For this review, take the finished solid that the model builds, in its own axes (mm). Face numbers are marked on the shaded views. A direction names the side the tool comes from. Round coordinates to 2 decimals unless told otherwise and drop trailing zeros. Write each loop counter-clockwise with the first axis right and the second up, starting at its lowest first coordinate (ties: lowest second). Pieces come first, ordered by that corner, then holes. Notation, with made-up numbers: (-25, 44.25) - (28, 44.25) arc R23 cw to (28, 55.25) - close; hole circle Ø1 at (85.5, 6.25). An arc over 180 degrees is marked (long way). One line per item, written item: value. Start each with the question number.
Q1. For probe 1 along Y at (x, z) = (0, 6.6); probe 2 along Y at (x, z) = (0, 1.5); probe 3 along Z at (x, y) = (1.75, -5.75), list the stretches that pass through material, from the lowest coordinate up.
Q2. Clearance check with flat-ended pins moving along their axes: pin 1 Ø2.5 at (x, y) = (-1.5, 1.5) entering from +Z; pin 2 Ø3.5 at (x, y) = (0, 0) entering from -Z; pin 3 Ø6 at (x, z) = (7, 1.5) entering from -Y; pin 4 Ø2 at (x, z) = (-6.5, 5.5) entering from +Y. State where each tip first meets the part, or that it passes through.
Q3. Add section D-D on x = -6.25. Write out the cut boundary in (y, z).
Q4. Add section C-C on z = 7.5. Write out the cut boundary in (x, y).
Q5. Add section A-A on y = 0. Write out the cut boundary in (x, z), and give its area (3 significant figures).
Q6. Mouldability with a two-part tool opening along X and no side actions: class the marked faces 1, 2 and 3 as +X half, -X half, draft (parallel to the pull), parting line (faces both ways), or undercut.
Q7. Tool access review of the marked faces 4 and 5: name each direction out of +Z, -Z, +X, -X, +Y, -Y from which nothing blocks a thin tool from reaching the whole face with its end or side.
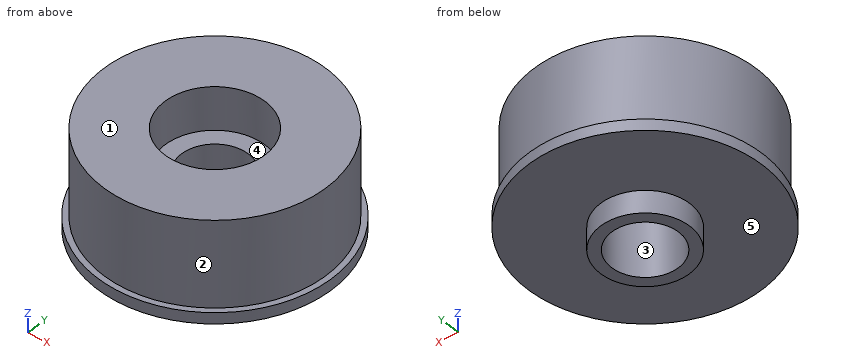
Autodesk Inventor part; units mm, degrees
ref_plane "YZ Plane" through (0, 0, 0) normal (1, 0, 0) x (0, 1, 0)
ref_plane "XZ Plane" through (0, 0, 0) normal (0, 1, 0) x (-1, 0, 0)
ref_plane "XY Plane" through (0, 0, 0) normal (0, 0, 1) x (1, 0, 0)
sketch "スケッチ1" plane through (0, 0, 0) normal (0, 0, 1) x (1, 0, 0)
  circle A0 centre (0, 0) radius 10 construction
  circle A1 centre (0, 0) radius 10.5 construction
  circle A2 centre (0, 0) radius 3 construction
  circle A3 centre (0, 0) radius 9.5 construction
  circle A4 centre (0, 0) radius 1.5
  dimension "d0" = 20
  dimension "d1" = 21
  dimension "d2" = 6
  dimension "d3" = 19
  dimension "d10" = 3
sketch "スケッチ2" plane through (0, 0, 0) normal (0, 0, 1) x (1, 0, 0)
  circle A0 centre (0, 0) radius 9.5 construction
  circle A1 centre (0, 0) radius 10 construction
  circle A2 centre (0, 0) radius 9.5
  circle A3 centre (0, 0) radius 10
extrude "押し出し1" add sketch "スケッチ2" along normal blind 8.75
sketch "スケッチ4" plane through (0, 0, 0) normal (0, 0, 1) x (1, 0, 0)
  circle A0 centre (0, 0) radius 3 construction
  circle A1 centre (0, 0) radius 9.5 construction
  circle A2 centre (0, 0) radius 9.5
  circle A3 centre (0, 0) radius 10
  circle A4 centre (0, 0) radius 3
extrude "押し出し3" add sketch "スケッチ4" along normal blind 8.75 contours A2 | A4
sketch "スケッチ6" plane through (0, 0, 0) normal (0, 0, 1) x (1, 0, 0)
  circle A0 centre (0, 0) radius 10 construction
  circle A1 centre (0, 0) radius 10.5 construction
  circle A2 centre (0, 0) radius 3 construction
  circle A3 centre (0, 0) radius 9.5 construction
  circle A4 centre (0, 0) radius 1.5
  circle A5 centre (0, 0) radius 10.5
  circle A6 centre (0, 0) radius 10
  circle A7 centre (0, 0) radius 10
  circle A8 centre (0, 0) radius 9.5
  circle A9 centre (0, 0) radius 3
  dimension "d15" = 20
  dimension "d16" = 21
  dimension "d17" = 6
  dimension "d18" = 19
  dimension "d19" = 3
extrude "押し出し6" add sketch "スケッチ6" along normal blind 1 contours A5
sketch "スケッチ7" plane through (0, 0, 0) normal (0, 0, 1) x (1, 0, 0)
  circle A0 centre (0, 0) radius 10 construction
  circle A1 centre (0, 0) radius 10.5 construction
  circle A2 centre (0, 0) radius 3 construction
  circle A3 centre (0, 0) radius 9.5 construction
  circle A4 centre (0, 0) radius 1.5
  circle A5 centre (0, 0) radius 10.5
  circle A6 centre (0, 0) radius 10
  circle A7 centre (0, 0) radius 9.5
  circle A8 centre (0, 0) radius 3
  circle A9 centre (0, 0) radius 4
  dimension "d22" = 20
  dimension "d23" = 21
  dimension "d24" = 6
  dimension "d25" = 19
  dimension "d26" = 3
  dimension "d27" = 8
extrude "押し出し7" add sketch "スケッチ7" against normal blind 2 contours A9
sketch "スケッチ8" plane through (0, 0, 0) normal (0, 0, 1) x (1, 0, 0)
  circle A0 centre (0, 0) radius 10 construction
  circle A1 centre (0, 0) radius 10.5 construction
  circle A2 centre (0, 0) radius 3 construction
  circle A3 centre (0, 0) radius 9.5 construction
  circle A4 centre (0, 0) radius 1.5
  circle A5 centre (0, 0) radius 10.5
  circle A6 centre (0, 0) radius 10
  circle A7 centre (0, 0) radius 9.5
  circle A8 centre (0, 0) radius 3
  circle A9 centre (0, 0) radius 4
  dimension "d30" = 20
  dimension "d31" = 21
  dimension "d32" = 6
  dimension "d33" = 19
  dimension "d34" = 3
  dimension "d35" = 8
extrude "押し出し8" cut sketch "スケッチ8" along normal blind 20 contours A4
sketch "スケッチ9" plane through (0, 0, 0) normal (0, 0, 1) x (1, 0, 0)
  circle A0 centre (0, 0) radius 10 construction
  circle A1 centre (0, 0) radius 10.5 construction
  circle A2 centre (0, 0) radius 3 construction
  circle A3 centre (0, 0) radius 9.5 construction
  circle A4 centre (0, 0) radius 1.5
  circle A5 centre (0, 0) radius 10.5
  circle A6 centre (0, 0) radius 10
  circle A7 centre (0, 0) radius 9.5
  circle A8 centre (0, 0) radius 3
  circle A9 centre (0, 0) radius 4
  dimension "d38" = 20
  dimension "d39" = 21
  dimension "d40" = 6
  dimension "d41" = 19
  dimension "d42" = 3
  dimension "d43" = 8
extrude "押し出し9" cut sketch "スケッチ9" along normal blind 20 contours A8
ref_plane "作業平面1" through (0, 0, 8.75) normal (0, 0, 1) x (1, 0, 0)
sketch "スケッチ10" plane through (0, 0, 8.75) normal (0, 0, 1) x (1, 0, 0)
  circle A0 centre (0, 0) radius 4.5
  dimension "d47" = 9
extrude "押し出し10" cut sketch "スケッチ10" against normal blind 3.85
properties part number "wheel"
Result set:
1. probe 1: y = -10 to -4.5, 4.5 to 10
1. probe 2: y = -10 to -3, 3 to 10
1. probe 3: z = 0 to 8.75
2. pin 1: stops at z = 4.9
2. pin 2: passes through
2. pin 3: stops at y = -9.69
2. pin 4: stops at y = 8.35
3. outline: (-8.44, 0) - (8.44, 0) - (8.44, 1) - (7.81, 1) - (7.81, 8.75) - (-7.81, 8.75) - (-7.81, 1) - (-8.44, 1) - close
4. outline: circle Ø20 at (0, 0); hole circle Ø9 at (0, 0)
5. outline: (-10.5, 0) - (-4, 0) - (-4, -2) - (-3, -2) - (-3, 4.9) - (-4.5, 4.9) - (-4.5, 8.75) - (-10, 8.75) - (-10, 1) - (-10.5, 1) - close; (3, -2) - (4, -2) - (4, 0) - (10.5, 0) - (10.5, 1) - (10, 1) - (10, 8.75) - (4.5, 8.75) - (4.5, 4.9) - (3, 4.9) - close
5. area: 116 mm^2
6. face 1: draft
6. face 2: parting line
6. face 3: undercut
7. face 4: +Z
7. face 5: -Z
